Build history of the part. All positions in model axes, mm. A direction names the side the tool comes from. Round coordinates to 2 decimals unless told otherwise and drop trailing zeros. Write each loop counter-clockwise with the first axis right and the second up, starting at its lowest first coordinate (ties: lowest second). Pieces come first, ordered by that corner, then holes. Notation, with made-up numbers: (31, 68) -> (88, 68) arc R29 ccw to (88, 102) -> close; hole circle Ø10 at (55.5, 22.25). An arc over 180 degrees is marked (long way). Return JSON: item names as keys, results as strings.
from build123d import *

# Parameters (mm, degrees)
F0_R     = 1
F0_R_2   = 2.05
F0_R_3   = 3.75
F0_R_4   = 6.25
F1_DEPTH = 1


with BuildPart() as f1:
    # F0 (on Top) → F1 (new body)
    with BuildSketch(Plane.XY):
        with BuildLine():
            Line((16.25, 9), (16.25, 10.5))
            ThreePointArc((16.25, 10.5), (14, 12.75), (11.75, 10.5))
            Line((11.75, 10.5), (11.75, 10))
            ThreePointArc((11.75, 10), (11.31066, 8.93934), (10.25, 8.5))
            Line((10.25, 8.5), (-14, 8.5))
            ThreePointArc((-14, 8.5), (-22.5, 0), (-14, -8.5))
            Line((-14, -8.5), (10.25, -8.5))
            ThreePointArc((10.25, -8.5), (11.31066, -8.93934), (11.75, -10))
            Line((11.75, -10), (11.75, -10.5))
            ThreePointArc((11.75, -10.5), (14, -12.75), (16.25, -10.5))
            Line((16.25, -10.5), (16.25, -9))
            ThreePointArc((16.25, -9), (16.501925, -8.16795), (17.173077, -7.615385))
            ThreePointArc((17.173077, -7.615385), (22.25, 0), (17.173077, 7.615385))
            ThreePointArc((17.173077, 7.615385), (16.501925, 8.16795), (16.25, 9))
        make_face()
        with Locations((-18.242641, -4.242641)):
            Circle(F0_R, mode=Mode.SUBTRACT)
        with Locations((-9.757359, -4.242641)):
            Circle(F0_R, mode=Mode.SUBTRACT)
        with Locations((14, -10.5)):
            Circle(F0_R, mode=Mode.SUBTRACT)
        with Locations((-14, 0)):
            Circle(F0_R_2, mode=Mode.SUBTRACT)
        with Locations((-18.242641, 4.242641)):
            Circle(F0_R, mode=Mode.SUBTRACT)
        with Locations((-9.757359, 4.242641)):
            Circle(F0_R, mode=Mode.SUBTRACT)
        with Locations((-1, 0)):
            Circle(F0_R_3, mode=Mode.SUBTRACT)
        with Locations((14, 0)):
            Circle(F0_R_4, mode=Mode.SUBTRACT)
        with Locations((14, 10.5)):
            Circle(F0_R, mode=Mode.SUBTRACT)
    extrude(amount=F1_DEPTH)


solid = f1.part
Q1. 3-axis set-ups, long thin cutter, end or side, ignore diameter. For faces 1 (the flat face through (-1.7, 8.5, 0.5)), 2 (the flat face through (16.25, 9.7, 0.5)), 3 (the flat face through (16.25, -9.8, 0.5)), 4 (the flat face through (-2, -8.5, 0.5)): which of +Z, -Z, +X, -X, +Y, -Y reach the whole face in a straight line?
Verdict:
{"face 1": "+Z, -Z, -X, +Y", "face 2": "+Z, -Z, +X, +Y", "face 3": "+Z, -Z, +X, -Y", "face 4": "+Z, -Z, -X, -Y"}
Q2. Saw through at C-C on x = 14. List the corners of the cut face in (y, z).
Verdict:
{"outline": "(-12.75, 0) -> (-11.5, 0) -> (-11.5, 1) -> (-12.75, 1) -> close; (-9.5, 0) -> (-6.25, 0) -> (-6.25, 1) -> (-9.5, 1) -> close; (6.25, 0) -> (9.5, 0) -> (9.5, 1) -> (6.25, 1) -> close; (11.5, 0) -> (12.75, 0) -> (12.75, 1) -> (11.5, 1) -> close"}
Q3. Pin check, flat tip, straight feed: pin 1 Ø6 at (x, y) = (-1, 0) entering from +Z. Stop position of the tip, or through.
Verdict:
{"pin 1": "passes through"}
Q4. Saw through at D-D on z = 0.65. Count the separate pieces of the cut face and the enclosed holes in it, then the cut area to 3 significant figures.
Verdict:
{"separate pieces": "1", "enclosed holes": "9", "area": "534 mm²"}
Q5. Saw through at B-B on y = 0. List the corners of the cut face in (x, z).
Verdict:
{"outline": "(-22.5, 0) -> (-16.05, 0) -> (-16.05, 1) -> (-22.5, 1) -> close; (-11.95, 0) -> (-4.75, 0) -> (-4.75, 1) -> (-11.95, 1) -> close; (2.75, 0) -> (7.75, 0) -> (7.75, 1) -> (2.75, 1) -> close; (20.25, 0) -> (22.25, 0) -> (22.25, 1) -> (20.25, 1) -> close"}
Q6. Saw through at A-A on x = -1. List the corners of the cut face in (y, z), then the cut area to 3 significant figures.
Verdict:
{"outline": "(-8.5, 0) -> (-3.75, 0) -> (-3.75, 1) -> (-8.5, 1) -> close; (3.75, 0) -> (8.5, 0) -> (8.5, 1) -> (3.75, 1) -> close", "area": "9.50 mm²"}
Q7. Wall check: L1, parallel to Y at x = 14, z = 0.7; L2, parallel to X at y = -1.75, z = 0.9; L3, parallel to Y at x = -1, z = 0.5. Give the ranges that are in metal, low to high.
Verdict:
{"L1": "y = -12.75 to -11.5, -9.5 to -6.25, 6.25 to 9.5, 11.5 to 12.75", "L2": "x = -22.32 to -15.07, -12.93 to -4.32, 2.32 to 8, 20 to 22.06", "L3": "y = -8.5 to -3.75, 3.75 to 8.5"}
